Autodesk Inventor part; units mm, degrees
ref_plane "YZ Plane" through (0, 0, 0) normal (1, 0, 0) x (0, 1, 0)
ref_plane "XZ Plane" through (0, 0, 0) normal (0, 1, 0) x (-1, 0, 0)
ref_plane "XY Plane" through (0, 0, 0) normal (0, 0, 1) x (1, 0, 0)
sketch "Sketch1" plane through (0, 0, 0) normal (0, 0, 1) x (1, 0, 0)
  line L0 (-49.5, 60.5) -> (49.5, 60.5)
  line L1 (49.5, 60.5) -> (49.5, -60.5)
  line L2 (49.5, -60.5) -> (-49.5, -60.5)
  line L3 (-49.5, -60.5) -> (-49.5, 60.5)
  line L4 (-49.5, 60.5) -> (49.5, -60.5) construction
  line L5 (49.5, 60.5) -> (-49.5, -60.5) construction
  point P0 (0, 0)
  dimension "d0" = 99
  dimension "d1" = 121
extrude "Extrusion1" add sketch "Sketch1" along normal blind 3
sketch "Sketch2" plane through (0, 0, 3) normal (0, 0, 1) x (1, 0, 0)
  line L0 (-47.3, 58.3) -> (47.3, 58.3)
  line L1 (47.3, 58.3) -> (47.3, -58.3)
  line L2 (47.3, -58.3) -> (-47.3, -58.3)
  line L3 (-47.3, -58.3) -> (-47.3, 58.3)
  line L4 (-47.3, 58.3) -> (47.3, -58.3) construction
  line L5 (47.3, 58.3) -> (-47.3, -58.3) construction
  point P0 (0, 0)
  dimension "d4" = 116.6
  dimension "d5" = 94.6
extrude "Extrusion2" add sketch "Sketch2" along normal blind 3
fillet "Fillet1" radius 2 4 edges at (49.5, 60.5, 1.5) (-49.5, 60.5, 1.5) (49.5, -60.5, 1.5) (-49.5, -60.5, 1.5)
sketch "Sketch5" plane through (0, 0, 6) normal (0, 0, 1) x (1, 0, 0)
  line L0 (44.3, -55.3) -> (-44.3, -55.3)
  line L1 (-44.3, -55.3) -> (-44.3, 55.3)
  line L2 (-44.3, 55.3) -> (44.3, 55.3)
  line L3 (44.3, 55.3) -> (44.3, -55.3)
  line L4 (44.3, -55.3) -> (-44.3, 55.3) construction
  line L5 (-44.3, -55.3) -> (44.3, 55.3) construction
  line L6 (47.3, 58.3) -> (-47.3, 58.3)
  line L7 (47.3, -58.3) -> (47.3, 58.3)
  line L8 (-78.6, 90.6) -> (-10, 90.6)
  line L9 (-10, 90.6) -> (-10, 20)
  line L10 (-10, 20) -> (-78.6, 20)
  line L11 (-78.6, 20) -> (-78.6, 90.6)
  line L12 (-78.6, 90.6) -> (-10, 20) construction
  line L13 (-10, 90.6) -> (-78.6, 20) construction
  line L14 (78.6, 90.6) -> (10, 90.6)
  line L15 (10, 90.6) -> (10, 20)
  line L16 (10, 20) -> (78.6, 20)
  line L17 (78.6, 20) -> (78.6, 90.6)
  line L18 (78.6, 90.6) -> (10, 20) construction
  line L19 (10, 90.6) -> (78.6, 20) construction
  line L20 (10, -20) -> (78.6, -20)
  line L21 (78.6, -20) -> (78.6, -90.6)
  line L22 (78.6, -90.6) -> (10, -90.6)
  line L23 (10, -90.6) -> (10, -20)
  line L24 (10, -20) -> (78.6, -90.6) construction
  line L25 (78.6, -20) -> (10, -90.6) construction
  line L26 (-78.6, -90.6) -> (-10, -90.6)
  line L27 (-10, -90.6) -> (-10, -20)
  line L28 (-10, -20) -> (-78.6, -20)
  line L29 (-78.6, -20) -> (-78.6, -90.6)
  line L30 (-78.6, -90.6) -> (-10, -20) construction
  line L31 (-10, -90.6) -> (-78.6, -20) construction
  point P0 (0, 0)
  point P1 (-10, -55.3)
  point P2 (-44.3, -20)
  point P3 (44.3, -20)
  point P4 (10, -55.3)
  point P5 (-44.3, 20)
  point P6 (-10, 55.3)
  point P7 (10, 55.3)
  point P8 (44.3, 20)
  dimension "d23" = 3
  dimension "d24" = 3
  dimension "d27" = 20
  dimension "d28" = 40
extrude "Extrusion5" cut sketch "Sketch5" against normal up to surface (3 mm away) contours L3 L20 L21 L22 L23 L0 | L0 L23 L20 L3 | L0 L27 L28 L1 L10 L9 L2 L15 L16 L3 L20 L23 | L27 L26 L29 L28 L1 L0 | L0 L1 L28 L27 | L16 L15 L2 L3 | L3 L2 L15 L6 L7 L16 | L7 L6 L15 L14 L17 L16 | L10 L11 L8 L9 L2 L1 | L1 L2 L9 L10
equation "\"BendRadius\" = Thickness"
equation "\"BendReliefWidth\" = Thickness"
equation "\"BendReliefDepth\" = 0.5 * Thickness"
equation "\"CornerReliefSize\" = 4 * Thickness"
equation "\"MinimumRemnant\" = 2 * Thickness"
equation "\"TransitionRadius\" = BendRadius"
equation "\"JacobiRadiusSize\" = BendRadius"
equation "\"GapSize\" = Thickness"
properties part number "_3DPrint"
Model file for the job. Use its own axes, mm. A direction names the side the tool comes from. Round coordinates to 2 decimals unless told otherwise and drop trailing zeros. Write each loop counter-clockwise with the first axis right and the second up, starting at its lowest first coordinate (ties: lowest second). Pieces come first, ordered by that corner, then holes. Notation, with made-up numbers: (82.5, 46.5) - (132.5, 46.5) arc R22 ccw to (132.5, 75.5) - close; hole circle Ø9 at (60.5, 71.5). An arc over 180 degrees is marked (long way). Use CSV: the item, a comma, the result in double quotes. Start each with the question number.
Item 1: Tool access for faces 4 (the face through (46, 20, 5)), 5 (the face through (0, -58.3, 4)), 6 (the face through (10, 57, 5)), 7 (the face through (0, 55.3, 5)), 8 (the face through (-10, -57, 5)): list every direction of +Z, -Z, +X, -X, +Y, -Y with a clear straight run to the whole face (end or side of a thin tool).
Item 2: Band-saw the part on A-A (z = 4.6). Write the cut outline in (x, y), and give its area (3 significant figures).
Item 3: Two-plate mould, pull along X, no slides. Class faces 1 (the face through (44.3, 0, 5)), 2 (the face through (0, 58.3, 4)), 3 (the face through (-10, 57, 5)): released by +X, released by -X, zero draft, split by the parting line, or undercut.
Item 4: Band-saw the part on B-B (y = 9). Write the cut outline in (x, z), and give its area (3 significant figures).
Item 5: Band-saw the part on C-C (x = 8.5). Write the cut outline in (y, z).
Item 6: Band-saw the part on D-D (y = 30.5). Write the cut outline in (x, z).
Item 7: Pin check, flat tips, straight feed: P1, Ø4, axis at x = 35.5, y = 8, coming from the +Z side; P2, Ø0.9, axis at y = -56, z = 5, coming from the -X side; P3, Ø0.9, axis at x = -2, z = 4, coming from the -Y side. Stop position of each tip, or through.
Item 8: Drill centre lines: L1, parallel to Y at x = 7, z = 3.7; L2, parallel to Z at x = 12.5, y = 48.5; L3, parallel to X at y = 17, z = 4.55. Where is each one in solid material? Low to high. Write a range as [from, to].
Checked values:
1,face 4,"+Z, +X, -X, +Y"
1,face 5,"+Z, +X, -X, -Y"
1,face 6,"+Z, +X, +Y, -Y"
1,face 7,"+Z, +X, -X"
1,face 8,"+Z, -X, +Y, -Y"
2,outline,"(-47.3, -20) - (-44.3, -20) - (-44.3, 20) - (-47.3, 20) - close; (-10, -58.3) - (10, -58.3) - (10, -55.3) - (-10, -55.3) - close; (-10, 55.3) - (10, 55.3) - (10, 58.3) - (-10, 58.3) - close; (44.3, -20) - (47.3, -20) - (47.3, 20) - (44.3, 20) - close"
2,area,"360 mm²"
3,face 1,"undercut"
3,face 2,"zero draft"
3,face 3,"released by -X"
4,outline,"(-49.5, 0) - (49.5, 0) - (49.5, 3) - (47.3, 3) - (47.3, 6) - (44.3, 6) - (44.3, 3) - (-44.3, 3) - (-44.3, 6) - (-47.3, 6) - (-47.3, 3) - (-49.5, 3) - close"
4,area,"315 mm²"
5,outline,"(-60.5, 0) - (60.5, 0) - (60.5, 3) - (58.3, 3) - (58.3, 6) - (55.3, 6) - (55.3, 3) - (-55.3, 3) - (-55.3, 6) - (-58.3, 6) - (-58.3, 3) - (-60.5, 3) - close"
6,outline,"(-49.5, 0) - (49.5, 0) - (49.5, 3) - (-49.5, 3) - close"
7,P1,"stops at z = 3"
7,P2,"stops at x = -10"
7,P3,"stops at y = -58.3"
8,L1,"y = [-58.3, -55.3], [55.3, 58.3]"
8,L2,"z = [0, 3]"
8,L3,"x = [-47.3, -44.3], [44.3, 47.3]"
